Check sheet for the modelled part. Datum: model origin and axes. Units: mm. Coordinates: 2 decimals unless noted, no trailing zeros. Use a Markdown table: item, result. Add a question column.
1) Go/stop test with flat-tipped pins: P1, Ø3, axis at x = 141.5, z = 4.5, coming from the -Y side; P2, Ø1.9, axis at y = 15, z = 2, coming from the +X side; P3, Ø1.9, axis at x = 14.5, z = 2, coming from the +Y side. Record where each tip stops, or that it passes through.
2) Sectioned sample at A-A, the plane z = 5.25. State how many separate pieces and enclosed holes the cut face has, then the cut area to 3 significant figures.
3) Thickness scan on line 1 (X direction, y = 9, z = 6); line 2 (X direction, y = 36.5, z = 2.25); line 3 (X direction, y = 65, z = 3.5). Record the ranges inside material, lowest first.
from build123d import *

# Parameters (mm, degrees)
SKETCH1_W           = 6.35
SKETCH1_H           = 25.4
SKETCH1_W_2         = 25.4
SKETCH1_H_2         = 6.35
BOSS_EXTRUDE1_DEPTH = 6.35
SKETCH2_R           = 3.175
CUT_EXTRUDE1_DEPTH  = 6.35
SKETCH3_R           = 3.175
CUT_EXTRUDE2_DEPTH  = 6.35


with BuildPart() as part:
    # Sketch1 → Boss-Extrude1 (new body)
    with BuildSketch(Plane.XY):
        with BuildLine():
            add(Edge.make_bspline(
                [(0, 171.45), (12.7, 88.9), (0, 6.35)],
                knots=[0, 0, 0, 1, 1, 1], degree=2))
            add(Edge.make_bspline(
                [(0, 6.35), (-3.175, -3.175), (6.35, 0)],
                knots=[0, 0, 0, 1, 1, 1], degree=2))
            add(Edge.make_bspline(
                [(6.35, 0), (88.9, 12.7), (171.45, 0)],
                knots=[0, 0, 0, 1, 1, 1], degree=2))
            add(Edge.make_bspline(
                [(177.8, 6.35), (180.975, -3.175), (171.45, 0)],
                knots=[0, 0, 0, 1, 1, 1], degree=2))
            add(Edge.make_bspline(
                [(177.8, 171.45), (165.1, 88.9), (177.8, 6.35)],
                knots=[0, 0, 0, 1, 1, 1], degree=2))
            add(Edge.make_bspline(
                [(171.45, 177.8), (180.975, 180.975), (177.8, 171.45)],
                knots=[0, 0, 0, 1, 1, 1], degree=2))
            add(Edge.make_bspline(
                [(6.35, 177.8), (88.9, 165.1), (171.45, 177.8)],
                knots=[0, 0, 0, 1, 1, 1], degree=2))
            add(Edge.make_bspline(
                [(0, 171.45), (-3.175, 180.975), (6.35, 177.8)],
                knots=[0, 0, 0, 1, 1, 1], degree=2))
        make_face()
        with Locations((15.875, 38.1)):
            Rectangle(SKETCH1_W, SKETCH1_H, mode=Mode.SUBTRACT)
        with Locations((38.1, 15.875)):
            Rectangle(SKETCH1_W_2, SKETCH1_H_2, mode=Mode.SUBTRACT)
        with Locations((15.875, 139.7)):
            Rectangle(SKETCH1_W, SKETCH1_H, mode=Mode.SUBTRACT)
        with Locations((161.925, 139.7)):
            Rectangle(SKETCH1_W, SKETCH1_H, mode=Mode.SUBTRACT)
        with Locations((139.7, 15.875)):
            Rectangle(SKETCH1_W_2, SKETCH1_H_2, mode=Mode.SUBTRACT)
        with Locations((161.925, 38.1)):
            Rectangle(SKETCH1_W, SKETCH1_H, mode=Mode.SUBTRACT)
    extrude(amount=BOSS_EXTRUDE1_DEPTH)

    # Sketch2 → Cut-Extrude1 (cut)
    with BuildSketch(Plane.XY.offset(6.35)):
        with Locations((69.85, 63.5)):
            Circle(SKETCH2_R)
    extrude(amount=-CUT_EXTRUDE1_DEPTH, mode=Mode.SUBTRACT)

    # Sketch3 → Cut-Extrude2 (cut)
    with BuildSketch(Plane.XY.offset(6.35)):
        with Locations((6.35, 6.35)):
            Circle(SKETCH3_R)
        with Locations((171.45, 6.35)):
            Circle(SKETCH3_R)
        with Locations((171.45, 171.45)):
            Circle(SKETCH3_R)
        with Locations((6.35, 171.45)):
            Circle(SKETCH3_R)
    extrude(amount=-CUT_EXTRUDE2_DEPTH, mode=Mode.SUBTRACT)


solid = part.part
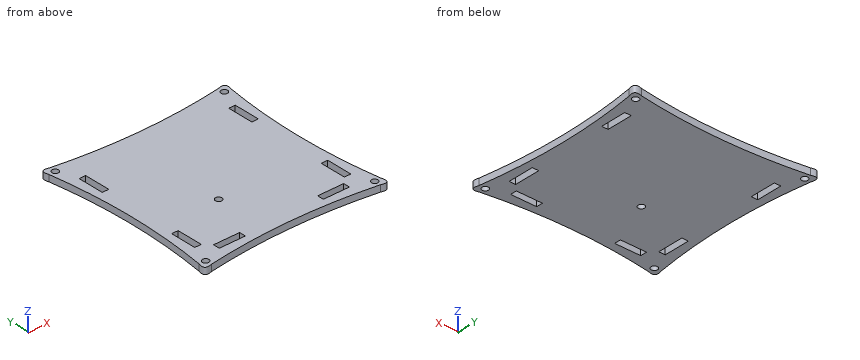
Solved:
| question | item | result |
|---|---|---|
| 1 | P1 | stops at y = 3.62 |
| 1 | P2 | stops at x = 176.67 |
| 1 | P3 | stops at y = 176.74 |
| 2 | separate pieces | 1 |
| 2 | enclosed holes | 11 |
| 2 | area | 27,700 mm2 |
| 3 | line 1 | x = 0.4 to 4.6, 8.1 to 169.7, 173.2 to 177.4 |
| 3 | line 2 | x = 3.79 to 12.7, 19.05 to 158.75, 165.1 to 174.01 |
| 3 | line 3 | x = 5.82 to 67.05, 72.65 to 171.98 |
